Check sheet for the modelled part. Datum: model origin and axes. Units: mm. A direction names the side the tool comes from. Give positions to 0.01 mm unless a question says otherwise; leave off trailing zeros. Order: outer loops, then holes, each group sorted by start corner. A loop starts at its lowest first (then second) coordinate and runs counter-clockwise, first axis right, second up. Notation, with made-up numbers: (34.25, -33.75) -> (78.25, -33.75) arc R26 ccw to (78.25, -5.75) -> close; hole circle Ø2 at (23, -34). An arc over 180 degrees is marked (long way). One line per question, with ' | ' between items. Start each with the question number.
from build123d import *

# Parameters (mm, degrees)
CROQUIS1_R               = 10
SALIENTE_EXTRUIR1_DEPTH  = 3
CROQUIS2_R               = 11.5
CROQUIS2_R_2             = 10
SALIENTE_EXTRUIR3_DEPTH  = 8
SALIENTE_EXTRUIR4_START  = 3
CROQUIS3_R               = 11.5
CROQUIS3_R_2             = 10
SALIENTE_EXTRUIR4_DEPTH  = 3
SALIENTE_EXTRUIR5_DEPTH  = 8
CROQUIS11_W              = 0.560242515
CROQUIS11_H              = 6
CORTAR_EXTRUIR3_DEPTH    = 8
CROQUIS12_W              = 2.5
CROQUIS12_H              = 0.622045166
SALIENTE_EXTRUIR6_DEPTH  = 3
CROQUIS13_W              = 5
CROQUIS13_H              = 50.27502784
SALIENTE_EXTRUIR7_DEPTH  = 8
CROQUIS15_W              = 2
CROQUIS15_H              = 50.27502784
CORTAR_EXTRUIR4_DEPTH    = 8
SALIENTE_EXTRUIR8_DEPTH  = 7
CROQUIS21_R              = 10
SALIENTE_EXTRUIR9_DEPTH  = 7
CROQUIS22_R              = 5
CORTAR_EXTRUIR5_DEPTH    = 30
CROQUIS23_R              = 10
SALIENTE_EXTRUIR10_DEPTH = 1.25
CORTAR_EXTRUIR6_START    = -1.5
CROQUIS24_R              = 10
CORTAR_EXTRUIR6_DEPTH    = 1.5
SALIENTE_EXTRUIR11_START = -3
CROQUIS25_R              = 13
SALIENTE_EXTRUIR11_DEPTH = 3
CORTAR_EXTRUIR14_START   = -10
CROQUIS30_R              = 10
CORTAR_EXTRUIR14_DEPTH   = 10
CROQUIS31_R              = 11.5
CROQUIS31_R_2            = 10
SALIENTE_EXTRUIR12_DEPTH = 7.75
CROQUIS32_R              = 10
SALIENTE_EXTRUIR13_DEPTH = 10.75
CROQUIS34_R              = 10
CORTAR_EXTRUIR15_DEPTH   = 7.75
CROQUIS36_R              = 3.825
SALIENTE_EXTRUIR14_DEPTH = 7.75
CROQUIS37_R              = 3.825
SALIENTE_EXTRUIR15_DEPTH = 9.5


with BuildPart() as part:
    # Croquis1 → Saliente-Extruir1 (new body)
    with BuildSketch(Plane.XY):
        Circle(CROQUIS1_R)
    extrude(amount=SALIENTE_EXTRUIR1_DEPTH)



with BuildPart() as body_2:
    # Croquis2 → Saliente-Extruir3 (new body)
    with BuildSketch(Plane.XY.offset(3)):
        Circle(CROQUIS2_R)
        Circle(CROQUIS2_R_2, mode=Mode.SUBTRACT)
    extrude(amount=SALIENTE_EXTRUIR3_DEPTH)


with BuildPart() as part_1:
    add(part.part)

    add(body_2.part)  # Saliente-Extruir4 merges body 2
    # Croquis3 → Saliente-Extruir4 (add)
    with BuildSketch(Plane(origin=(0, 0, 3), x_dir=(-1, 0, 0), z_dir=(0, 0, -1)).offset(SALIENTE_EXTRUIR4_START)):
        with Locations(Location((0, 0, 0), (0, 0, 180))):
            Circle(CROQUIS3_R)
        with Locations(Location((0, 0, 0), (0, 0, 180))):
            Circle(CROQUIS3_R_2, mode=Mode.SUBTRACT)
    extrude(amount=-SALIENTE_EXTRUIR4_DEPTH)

    # Croquis12 → Saliente-Extruir6 (add)
    with BuildSketch(Plane.XY.offset(3)):
        with Locations((-1.25, -11.188977417)):
            Rectangle(CROQUIS12_W, CROQUIS12_H)
        with Locations((1.25, -11.188977417)):
            Rectangle(CROQUIS12_W, CROQUIS12_H)
        Polygon((2.5, -11.5), (2.5, -61.5), (-2.5, -61.5), (-2.5, -11.5), (0, -11.5), align=None)
    extrude(amount=-SALIENTE_EXTRUIR6_DEPTH)

    # Croquis13 → Saliente-Extruir7 (add)
    with BuildSketch(Plane.XY.offset(3)):
        with Locations((0, -36.36248608)):
            Rectangle(CROQUIS13_W, CROQUIS13_H)
    extrude(amount=SALIENTE_EXTRUIR7_DEPTH)

    # Croquis15 → Cortar-Extruir4 (cut)
    with BuildSketch(Plane(origin=(2.5, 0, 0), x_dir=(0, 0, -1), z_dir=(1, 0, 0))):
        with Locations((-10, -36.36248608)):
            Rectangle(CROQUIS15_W, CROQUIS15_H)
        with Locations((-1, -36.36248608)):
            Rectangle(CROQUIS15_W, CROQUIS15_H)
    extrude(amount=-CORTAR_EXTRUIR4_DEPTH, mode=Mode.SUBTRACT)

    # Croquis16 → Saliente-Extruir8 (add)
    with BuildSketch(Plane.XY.offset(9)):
        Polygon((-2.5, -61.5), (-3.5, -61.5), (-3.5, -10.232955502), (3.5, -10.232955502), (3.5, -61.5), (2.5, -61.5), align=None)
    extrude(amount=-SALIENTE_EXTRUIR8_DEPTH)

    # Croquis21 → Saliente-Extruir9 (add)
    with BuildSketch(Plane(origin=(0, 0, 2), x_dir=(-1, 0, 0), z_dir=(0, 0, -1))):
        with Locations((0, -52.72497216)):
            Circle(CROQUIS21_R)
    extrude(amount=-SALIENTE_EXTRUIR9_DEPTH)

    # Croquis22 → Cortar-Extruir5 (cut)
    with BuildSketch(Plane(origin=(0, 0, 2), x_dir=(-1, 0, 0), z_dir=(0, 0, -1))):
        with Locations((0, -52.72497216)):
            Circle(CROQUIS22_R)
    extrude(amount=-CORTAR_EXTRUIR5_DEPTH, mode=Mode.SUBTRACT)

    # Croquis23 → Saliente-Extruir10 (add)
    with BuildSketch(Plane.XY.offset(11)):
        with BuildLine():
            Line((-2.5, -11.22497216), (2.5, -11.22497216))
            ThreePointArc((2.5, -11.22497216), (0, 11.5), (-2.5, -11.22497216))
        make_face()
        Circle(CROQUIS23_R, mode=Mode.SUBTRACT)
    extrude(amount=SALIENTE_EXTRUIR10_DEPTH)

    # Croquis24 → Cortar-Extruir6 (cut)
    with BuildSketch(Plane.XY.offset(12.25).offset(CORTAR_EXTRUIR6_START)):
        with BuildLine():
            Line((-2.5, -11.22497216), (2.5, -11.22497216))
            ThreePointArc((2.5, -11.22497216), (0, 11.5), (-2.5, -11.22497216))
        make_face()
        Circle(CROQUIS24_R, mode=Mode.SUBTRACT)
    extrude(amount=CORTAR_EXTRUIR6_DEPTH, mode=Mode.SUBTRACT)

    # Croquis25 → Saliente-Extruir11 (add)
    with BuildSketch(Plane.XY.offset(10.75).offset(SALIENTE_EXTRUIR11_START)):
        Circle(CROQUIS25_R)
        with BuildLine():
            ThreePointArc((2.5, -11.22497216), (0, 11.5), (-2.5, -11.22497216))
            Line((-2.5, -11.22497216), (2.5, -11.22497216))
        make_face(mode=Mode.SUBTRACT)
    extrude(amount=SALIENTE_EXTRUIR11_DEPTH)

    # Croquis30 → Cortar-Extruir14 (cut)
    with BuildSketch(Plane.XY.offset(3).offset(CORTAR_EXTRUIR14_START)):
        Circle(CROQUIS30_R)
    extrude(amount=CORTAR_EXTRUIR14_DEPTH, mode=Mode.SUBTRACT)

    # Croquis31 → Saliente-Extruir12 (add)
    with BuildSketch(Plane(origin=(0, 0, 0), x_dir=(-1, 0, 0), z_dir=(0, 0, -1))):
        with Locations(Location((0, 0, 0), (0, 0, 180))):
            Circle(CROQUIS31_R)
        with Locations(Location((0, 0, 0), (0, 0, 180))):
            Circle(CROQUIS31_R_2, mode=Mode.SUBTRACT)
    extrude(amount=-SALIENTE_EXTRUIR12_DEPTH)

    # Croquis32 → Saliente-Extruir13 (add)
    with BuildSketch(Plane(origin=(0, 0, 0), x_dir=(-1, 0, 0), z_dir=(0, 0, -1))):
        Circle(CROQUIS32_R)
    extrude(amount=-SALIENTE_EXTRUIR13_DEPTH)

    # Croquis34 → Cortar-Extruir15 (cut)
    with BuildSketch(Plane.XY.offset(10.75)):
        Circle(CROQUIS34_R)
    extrude(amount=-CORTAR_EXTRUIR15_DEPTH, mode=Mode.SUBTRACT)

    # Croquis36 → Saliente-Extruir14 (add)
    with BuildSketch(Plane.XY.offset(3)):
        Circle(CROQUIS36_R)
    extrude(amount=SALIENTE_EXTRUIR14_DEPTH)

    # Croquis37 → Saliente-Extruir15 (add)
    with BuildSketch(Plane.XY.offset(10.75)):
        Circle(CROQUIS37_R)
    extrude(amount=SALIENTE_EXTRUIR15_DEPTH)


with BuildPart() as body_2_2:
    # Croquis9 → Saliente-Extruir5 (new body)
    with BuildSketch(Plane.XY.offset(11)):
        Polygon((11.5, 0), (11.5, 3), (12.060242515, 3), (12.060242515, -3), (11.5, -3), align=None)
    extrude(amount=-SALIENTE_EXTRUIR5_DEPTH)

    # Croquis11 → Cortar-Extruir3 (cut)
    with BuildSketch(Plane.XY.offset(11)):
        with Locations((11.780121257, 0)):
            Rectangle(CROQUIS11_W, CROQUIS11_H)
    extrude(amount=-CORTAR_EXTRUIR3_DEPTH, mode=Mode.SUBTRACT)


solid = part_1.part
1. Tool access check on faces 1 (the face through (-1, 12, 7.75)), 2 (the face through (0, 0, 20.25)), 3 (the face through (-2.17, -9.76, 6.93)). Record the directions out of +Z, -Z, +X, -X, +Y, -Y that give a thin tool (end or side, any length) a straight path to the whole face; none if there is none.
2. Cross-section at A-A on z = 5.75. Record the boundary of the cut face in (x, y) (3 decimals).
3. Cross-section at B-B on x = 0. Record the boundary of the cut face in (y, z) (3 decimals).
4. Cross-section at D-D on z = 18.25. Record the boundary of the cut face in (x, y) (3 decimals), and give its area (3 significant figures).
5. Scan lines: probe 1 along Z at (x, y) = (5, -46); probe 2 along Y at (x, z) = (-0.25, 12.5); probe 3 along X at (y, z) = (-40.5, 6.5). Record each from-to range of solid material in increasing order.
6. Go/stop test with flat-tipped pins: pin 1 (10 mm diameter, centred on x = -9, z = 9, fed in from +Y); pin 2 (3.5 mm diameter, centred on y = -21, z = 6, fed in from -X); pin 3 (10 mm diameter, centred on y = -24, z = 6, fed in from +X); pin 4 (1 mm diameter, centred on x = -8.5, y = -45.5, fed in from -Z). Record where each tip stops, or that it passes through.
7. Cross-section at C-C on y = 0. Record the boundary of the cut face in (x, z) (3 decimals).
8. Mould release check, pull along Y, two halves, no side actions. Record for faces 4 (the face through (0.39, -62.717, 5.451)), 5 (the face through (0, -43, 9)): +Y half, -Y half, draft (parallel to the pull), parting line (faces both ways), or undercut.
Response values:
1) face 1: -Z | face 2: +Z, +X, -X, +Y, -Y | face 3: +Z
2) outline: circle Ø7.65 at (0, 0); (-3.5, -43.357) arc R10 ccw (long way) to (3.5, -43.357) -> (3.5, -10.954) arc R11.5 ccw (long way) to (-3.5, -10.954) -> close; hole circle Ø20 at (0, 0); hole circle Ø10 at (0, -52.725)
3) outline: (-62.725, 2) -> (-57.725, 2) -> (-57.725, 9) -> (-62.725, 9) -> close; (-47.725, 2) -> (-11.5, 2) -> (-11.5, 0) -> (11.5, 0) -> (11.5, 7.75) -> (13, 7.75) -> (13, 10.75) -> (10, 10.75) -> (10, 3) -> (3.825, 3) -> (3.825, 20.25) -> (-3.825, 20.25) -> (-3.825, 3) -> (-10, 3) -> (-10, 10.75) -> (-13, 10.75) -> (-13, 9) -> (-47.725, 9) -> close
4) outline: circle Ø7.65 at (0, 0) | area: 46.0 mm²
5) probe 1: z = 2 to 9 | probe 2: y = -3.82 to 3.82 | probe 3: x = -3.5 to 3.5
6) pin 1: stops at y = 12.37 | pin 2: stops at x = -3.5 | pin 3: stops at x = 3.5 | pin 4: passes through
7) outline: (-13, 7.75) -> (-11.5, 7.75) -> (-11.5, 0) -> (11.5, 0) -> (11.5, 7.75) -> (13, 7.75) -> (13, 10.75) -> (10, 10.75) -> (10, 3) -> (3.825, 3) -> (3.825, 20.25) -> (-3.825, 20.25) -> (-3.825, 3) -> (-10, 3) -> (-10, 10.75) -> (-13, 10.75) -> close
8) face 4: undercut | face 5: draft
